Geometry check sheet. Reference: the model listing, model coordinates, mm. Give positions to 0.01 mm unless a question says otherwise; leave off trailing zeros. Order: outer loops, then holes, each group sorted by start corner. A loop starts at its lowest first (then second) coordinate and runs counter-clockwise, first axis right, second up. Notation, with made-up numbers: M 34,86.5 L 53,86.5 A12 cw 53,105.5 Z; hole C 35.25,32.5 d10. An arc over 180 degrees is marked long. Answer as CSV lines item,"result". Start each with the question number.
```python
from build123d import *

# Parameters (mm, degrees)
SKETCH5_R           = 5
BOSS_EXTRUDE1_DEPTH = 10
SKETCH7_R           = 5
BOSS_EXTRUDE2_DEPTH = 20


with BuildPart() as part:
    # Sketch5 → Boss-Extrude1 (new body)
    with BuildSketch(Plane(origin=(0, 0, 0), x_dir=(1, 0, 0), z_dir=(0, 1, 0))):
        with BuildLine():
            Line((-425, 10), (425, 10))
            ThreePointArc((425, 10), (435, 0), (425, -10))
            Line((425, -10), (-425, -10))
            ThreePointArc((-425, -10), (-435, 0), (-425, 10))
        make_face()
        with Locations((-425, 0)):
            Circle(SKETCH5_R, mode=Mode.SUBTRACT)
    extrude(amount=-BOSS_EXTRUDE1_DEPTH)

    # Sketch7 → Boss-Extrude2 (add)
    with BuildSketch(Plane(origin=(0, 0, 0), x_dir=(1, 0, 0), z_dir=(0, 1, 0))):
        with Locations((425, 0)):
            Circle(SKETCH7_R)
    extrude(amount=BOSS_EXTRUDE2_DEPTH)


solid = part.part
```
Item 1: Section check B-B on y = 6. Record the boundary of the cut face in (x, z), then the cut area to 3 significant figures.
Item 2: Scan lines: line 1 along Z through (x, y) = (-425, -4.75); line 2 along X through (y, z) = (-3.75, 0); line 3 along X through (y, z) = (13, 1). Record each from-to range of solid material in increasing order.
Item 3: Section check C-C on x = -320.5. Record the boundary of the cut face in (y, z).
Item 4: Section check A-A on z = 0. Record the boundary of the cut face in (x, y).
Item 5: Depth check by flat-ended pin: pin 1 Ø1.5 at (y, z) = (11.5, -6.5) entering from +X; pin 2 Ø3 at (x, z) = (-135.5, -6) entering from +Y; pin 3 Ø8 at (y, z) = (10.5, 6) entering from +X; pin 4 Ø5 at (y, z) = (9.5, -3.5) entering from +X. Enter the tip coordinate at first touch or a pass-through.
Numbers:
1,outline,"C 425,0 d10"
1,area,"78.5 mm2"
2,line 1,"-10 to -5, 5 to 10"
2,line 2,"-435 to -430, -420 to 435"
2,line 3,"420.1 to 429.9"
3,outline,"M -10,-10 L 0,-10 L 0,10 L -10,10 Z"
4,outline,"M -435,-10 L -430,-10 L -430,0 L -435,0 Z; M -420,-10 L 435,-10 L 435,0 L 430,0 L 430,20 L 420,20 L 420,0 L -420,0 Z"
5,pin 1,"through"
5,pin 2,"y = 0"
5,pin 3,"x = 429.58"
5,pin 4,"x = 429.9"
